Geometry: final body of the model. Coordinates: model frame, mm. Face numbers are marked on the shaded views. A direction names the side the tool comes from. Round coordinates to 2 decimals unless told otherwise and drop trailing zeros. Loops run counter-clockwise (first coordinate to the right, second up) from the corner with the lowest first, then second, coordinate; pieces in that order, holes last. Notation, with made-up numbers: M 20,45 L 69,45 A25 ccw 69,78 Z; hole C -7,-21.75 d4. An arc over 180 degrees is marked long. Answer as a JSON object with one key per item and string values.
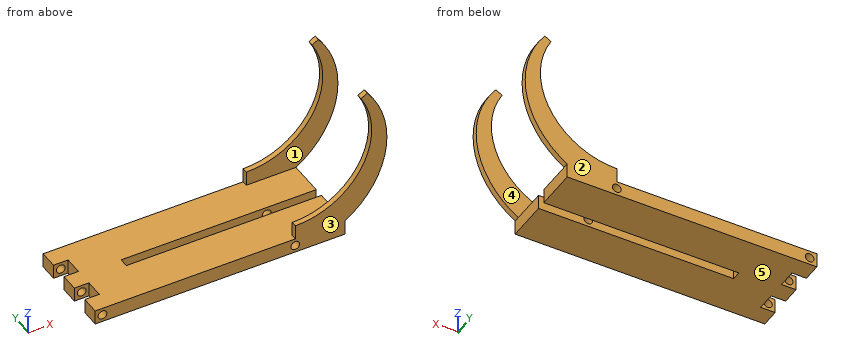
```python
from build123d import *

# Parameters (mm, degrees)
PAD_DEPTH           = 4
SKETCH001_R         = 1.2
POCKET_DEPTH        = 25.001
PAD001_DEPTH        = 1.5
LINEARPATTERN_COUNT = 2
LINEARPATTERN_PITCH = 23.5
SKETCH003_R         = 1.2
POCKET001_DEPTH     = 25.001
SKETCH004_W         = 57.256356
SKETCH004_H         = 2.5
POCKET002_DEPTH     = 40.745142


with BuildPart() as part:
    # Sketch → Pad (new body)
    with BuildSketch(Plane.XY):
        Polygon((41.369523, 12.5), (-27.256356, 12.5), (-27.256356, 7.5), (-23.256356, 7.5), (-23.256356, 2.5), (-27.256356, 2.5), (-27.256356, -2.5), (-23.256356, -2.5), (-23.256356, -7.5), (-27.256356, -7.5), (-27.256356, -12.5), (41.369523, -12.5), align=None)
    extrude(amount=PAD_DEPTH)

    # Sketch001 → Pocket (cut, through all)
    with BuildSketch(Plane.XZ.offset(12.5)):
        with Locations((-25.256356, 2)):
            Circle(SKETCH001_R)
    extrude(amount=-POCKET_DEPTH, mode=Mode.SUBTRACT)

    # Sketch002 → Pad001 (new body)
    with BuildSketch(Plane.XZ.offset(12.5)):
        with BuildLine():
            ThreePointArc((27.743644, 8), (45.994413, 18.612054), (45.799645, 39.722912))
            Line((47.519264, 40.744142), (45.799645, 39.722912))
            ThreePointArc((27.743644, 0), (50.388512, 14.180292), (47.519264, 40.744142))
            Line((27.743644, 8), (27.743644, 0))
        make_face()
    pad001 = extrude(amount=-PAD001_DEPTH)

    # LinearPattern: Pad001 ×2
    with Locations(*[(0, i * LINEARPATTERN_PITCH, 0) for i in range(1, LINEARPATTERN_COUNT)]):
        add(pad001)

    # Sketch003 → Pocket001 (cut, through all)
    with BuildSketch(Plane(origin=(0, 12.5, 0), x_dir=(-1, 0, 0), z_dir=(0, 1, 0))):
        with Locations((-27.743644, 2)):
            Circle(SKETCH003_R)
    extrude(amount=-POCKET001_DEPTH, mode=Mode.SUBTRACT)

    # Sketch004 → Pocket002 (cut, through all)
    with BuildSketch(Plane(origin=(0, 0, 0), x_dir=(1, 0, 0), z_dir=(0, 0, -1))):
        with Locations((16.371822, 0)):
            Rectangle(SKETCH004_W, SKETCH004_H)
    extrude(amount=-POCKET002_DEPTH, mode=Mode.SUBTRACT)


solid = part.part
```
1) Cut plane A-A on x = 19. Return the cut outline in (y, z), and give its area (3 significant figures).
Geometry results:
{"outline": "M -12.5,0 L -1.25,0 L -1.25,4 L -12.5,4 Z; M 1.25,0 L 12.5,0 L 12.5,4 L 1.25,4 Z", "area": "90.0 mm2"}
2) Cut plane C-C on z = 11. Return the cut outline in (x, y), and give its area (3 significant figures).
Geometry results:
{"outline": "M 38.56,-12.5 L 48.55,-12.5 L 48.55,-11 L 38.56,-11 Z; M 38.56,11 L 48.55,11 L 48.55,12.5 L 38.56,12.5 Z", "area": "30.0 mm2"}
3) Cut plane B-B on y = -0.5. Return the cut outline in (x, z), and give its area (3 significant figures).
Geometry results:
{"outline": "M -27.26,0 L -12.26,0 L -12.26,4 L -27.26,4 Z; hole C -25.26,2 d2.4", "area": "55.5 mm2"}
4) Line query: probe 1 along Y at (x, z) = (49, 14); probe 2 along Z at (x, y) = (9, -4); probe 3 along X at (y, z) = (11.5, 38). Output: solid intervals per line, ascending.
Geometry results:
{"probe 1": "-12.5 to -11, 11 to 12.5", "probe 2": "0 to 4", "probe 3": "46.72 to 49.4"}
5) First-contact query: pin 1 (4 mm diameter, centred on x = -18, y = -5.5, fed in from +Z); pin 2 (3 mm diameter, centred on y = 4.5, z = 3, fed in from +X); pin 3 (0.8 mm diameter, centred on y = -12, z = 6.5, fed in from -X); pin 4 (4 mm diameter, centred on x = 27.74, z = 2, fed in from -Y). Flat tips, straight axial feed; report the tip coordinate or a pass-through.
Geometry results:
{"pin 1": "z = 4", "pin 2": "x = 41.37", "pin 3": "x = 27.74", "pin 4": "y = -12.5"}
6) Pull-direction query (Y, two-part tool) for the marked faces 1, 2 and 3; classes: +Y half, -Y half, draft (parallel to the pull), parting line (faces both ways), or undercut.
Geometry results:
{"face 1": "undercut", "face 2": "+Y half", "face 3": "-Y half"}
7) Set-up query: the marked faces 4 and 5. Return all of +Z, -Z, +X, -X, +Y, -Y with unobstructed straight access to the full face (end or side cutting, diameter ignored); none if empty.
Geometry results:
{"face 4": "+Z, +X, -X", "face 5": "-Z, +X, -X, +Y, -Y"}
8) Cut plane D-D on y = -9. Return the cut outline in (x, z).
Geometry results:
{"outline": "M -27.26,0 L 41.37,0 L 41.37,4 L -27.26,4 Z; hole C -25.26,2 d2.4; hole C 27.74,2 d2.4"}
